The figure shows three views and two pictorial views of one solid part (mm, origin at its lowest corner). Answer the questions. A direction names the side the tool comes from. Round coordinates to 2 decimals unless told otherwise and drop trailing zeros. Order: outer loops, then holes, each group sorted by start corner. A loop starts at its lowest first (then second) coordinate and runs counter-clockwise, first axis right, second up. Notation, with made-up numbers: M -14.5,72.5 L -10.5,72.5 A23 cw -10.5,91.5 Z; hole C 77.25,60 d1. An arc over 180 degrees is marked long. Answer as CSV lines item,"result".
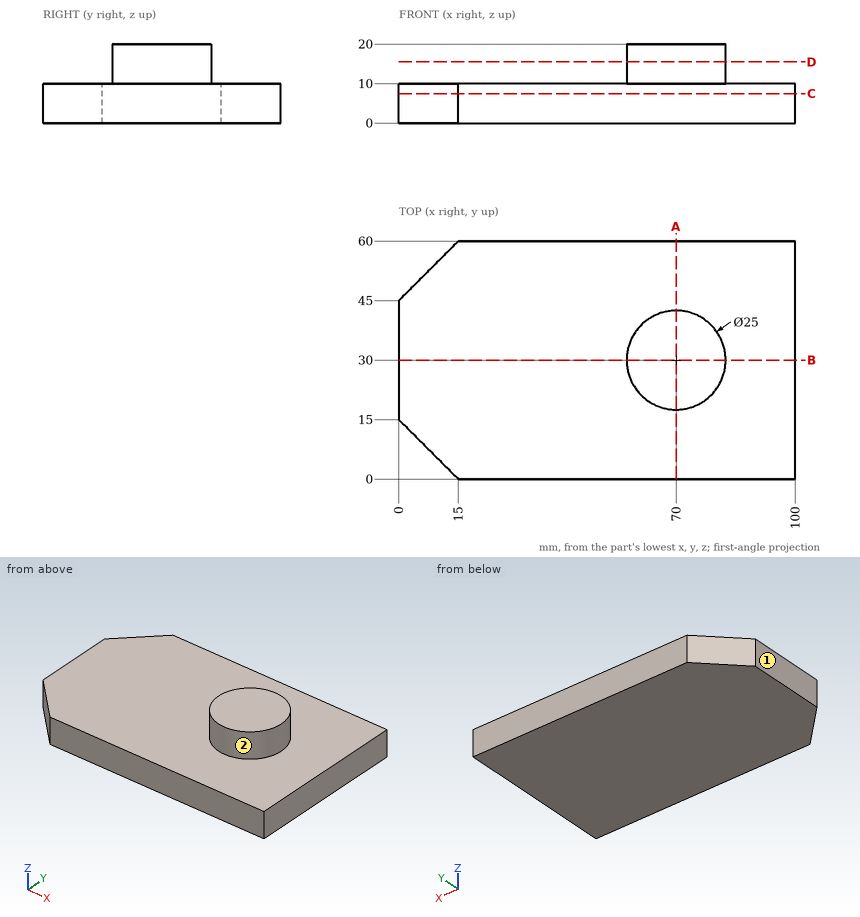
Item 1: A cutting plane is placed at C-C, the plane z = 7.5. Determine the outline of the cut face in (x, y), and give its area (4 significant figures).
Ans:
outline,"M 0,15 L 15,0 L 100,0 L 100,60 L 15,60 L 0,45 Z"
area,"5,775 mm2"
Item 2: Flat-ended cylindrical pins translate along their axes: pin 1 (8 mm diameter, centred on x = 24.5, z = 16, fed in from -Y); pin 2 (10 mm diameter, centred on x = 67, y = 53.5, fed in from +Z). Find the tip coordinate at first contact, or state that the pin passes through.
Ans:
pin 1,"through"
pin 2,"z = 10"
Item 3: A cutting plane is placed at A-A, the plane x = 70. Determine the outline of the cut face in (y, z), and give its area (3 significant figures).
Ans:
outline,"M 0,0 L 60,0 L 60,10 L 42.5,10 L 42.5,20 L 17.5,20 L 17.5,10 L 0,10 Z"
area,"850 mm2"
Item 4: A tool of negligible diameter and unlimited length cuts with its end or side. For the marked faces 1 and 2, from which of +Z, -Z, +X, -X, +Y, -Y can it reach the whole face along a straight path? Write none if from no direction.
Ans:
face 1,"+Z, -Z, -X, +Y, -Y"
face 2,"+Z"
Item 5: A cutting plane is placed at D-D, the plane z = 15.5. Determine the outline of the cut face in (x, y), and give its area (3 significant figures).
Ans:
outline,"C 70,30 d25"
area,"491 mm2"
Item 6: A cutting plane is placed at B-B, the plane y = 30. Determine the outline of the cut face in (x, z), and give its area (3 significant figures).
Ans:
outline,"M 0,0 L 100,0 L 100,10 L 82.5,10 L 82.5,20 L 57.5,20 L 57.5,10 L 0,10 Z"
area,"1,250 mm2"
Item 7: Find the intervals of material crossed by probe 1 along Z at (x, y) = (18, 7.5); probe 2 along X at (y, z) = (30.5, 13.75); probe 3 along X at (y, z) = (41, 15), in increasing order. Write a range as [from, to].
Ans:
probe 1,"[0, 10]"
probe 2,"[57.51, 82.49]"
probe 3,"[64.06, 75.94]"
